from build123d import *

# Parameters (mm, degrees)
F0_W     = 50.8
F0_H     = 0.7874
F3_R     = 3.3655
F4_DEPTH = 25.4


with BuildPart() as f2:
    # F2: sweep along a path in F1
    with BuildLine(Plane.YZ) as f2_path:
        Line((0, 0), (0, 127))
        ThreePointArc((0, 127), (-5.3913965951, 151.3190184681), (-20.5553226245, 171.0810316215))
        ThreePointArc((-20.5553226245, 171.0810316215), (-25.9637465294, 174.5265776491), (-32.0796557913, 176.4549164323))
        Line((-32.0796557913, 176.4549164323), (-63.9523993907, 182.0749410781))
    # F0 (on Top) → F2 (sweep)
    with BuildSketch(Plane.XY):
        Rectangle(F0_W, F0_H)
    sweep(path=f2_path.line)

    # F3 (on face) → F4 (cut)
    with BuildSketch(Plane(origin=(0, 29.2766132085, 166.0359242292), x_dir=(1, 0, 0), z_dir=(0, 0.1736481777, 0.984807753))):
        with Locations((-9.525, -78.7228004607)):
            Circle(F3_R)
        with Locations((9.525, -78.7228004607)):
            Circle(F3_R)
    extrude(amount=-F4_DEPTH, mode=Mode.SUBTRACT)


solid = f2.part
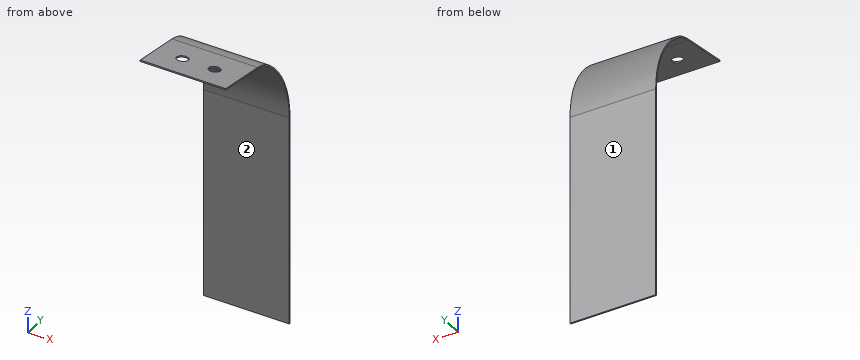
Read the model definition and answer for the solid it produces. Units are mm, in the model's axes. Face numbers are marked on the shaded views. A direction names the side the tool comes from. Give positions to 0.01 mm unless a question says otherwise; leave off trailing zeros. Loops run counter-clockwise (first coordinate to the right, second up) from the corner with the lowest first, then second, coordinate; pieces in that order, holes last. Notation, with made-up numbers: (-11, 7.5) -> (29, 7.5) arc R19 ccw to (29, 24.5) -> close; hole circle Ø1 at (81.25, 26.5). An arc over 180 degrees is marked (long way). Answer as CSV lines item,"result".
Item 1: Consider line 1 (Y direction, x = 13, z = 46.5); line 2 (Z direction, x = -18.5, y = -32); line 3 (Y direction, x = -12, z = 140). Determine where each line is inside the solid, lowest interval first. Write a range as [from, to].
Returned:
line 1,"y = [-0.39, 0.39]"
line 2,"z = [176.04, 176.84]"
line 3,"y = [-1.89, -1.08]"
Item 2: Each of these flat-tipped pins is pushed along its axis until it touches: pin 1 (4 mm diameter, centred on x = -13.5, z = 133, fed in from -Y); pin 2 (5 mm diameter, centred on x = 7, y = -11, fed in from -Z); pin 3 (10 mm diameter, centred on x = 9.5, y = -13.5, fed in from +Z). Where does it stop, or does it pass through?
Returned:
pin 1,"stops at y = -0.96"
pin 2,"stops at z = 156.34"
pin 3,"stops at z = 169.81"
Item 3: Find section D-D on y = -27.5. Give the vertices of the cut face in (x, z).
Returned:
outline,"(-25.4, 174.76) -> (25.4, 174.76) -> (25.4, 175.6) -> (-25.4, 175.6) -> close"
Item 4: For the marked faces 1 and 2, determine the directions among +Z, -Z, +X, -X, +Y, -Y from which every point of the face is accessible in a straight line to the end or side of a thin tool.
Returned:
face 1,"+Z, -Z, +X, -X, +Y"
face 2,"-Z, +X, -X, -Y"
Item 5: Find section A-A on x = -9. Give the vertices of the cut face in (y, z).
Returned:
outline,"(-64.02, 181.69) -> (-51.66, 179.51) -> (-51.52, 180.28) -> (-63.88, 182.46) -> close; (-45.11, 178.35) -> (-32.15, 176.07) arc R24.17 cw to (-20.81, 170.78) arc R57.15 cw to (-0.39, 127) -> (-0.39, 0) -> (0.39, 0) -> (0.39, 127) arc R57.94 ccw to (-20.3, 171.38) arc R24.96 ccw to (-32.01, 176.84) -> (-44.98, 179.13) -> close"
Item 6: Find section B-B on x = 8. Give the vertices of the cut face in (y, z).
Returned:
outline,"(-64.02, 181.69) -> (-51.34, 179.45) -> (-51.2, 180.23) -> (-63.88, 182.46) -> close; (-45.43, 178.41) -> (-32.15, 176.07) arc R24.17 cw to (-20.81, 170.78) arc R57.15 cw to (-0.39, 127) -> (-0.39, 0) -> (0.39, 0) -> (0.39, 127) arc R57.94 ccw to (-20.3, 171.38) arc R24.96 ccw to (-32.01, 176.84) -> (-45.3, 179.19) -> close"
Item 7: Find section C-C on z = 123. Give the vertices of the cut face in (x, y).
Returned:
outline,"(-25.4, -0.39) -> (25.4, -0.39) -> (25.4, 0.39) -> (-25.4, 0.39) -> close"
